Read the model definition and answer for the solid it produces. Units are mm, in the model's axes. Face numbers are marked on the shaded views. A direction names the side the tool comes from. Round coordinates to 2 decimals unless told otherwise and drop trailing zeros. Order: outer loops, then holes, each group sorted by start corner. A loop starts at its lowest first (then second) coordinate and runs counter-clockwise, first axis right, second up. Notation, with made-up numbers: (67.5, 10) -> (119.5, 10) arc R6 cw to (119.5, 14) -> close; hole circle Ø1 at (88, 74). An arc over 180 degrees is marked (long way). Answer as a JSON object with one key per item and string values. Group by question number.
Item 1: Consider probe 1 along X at (y, z) = (2.5, 4); probe 2 along Z at (x, y) = (0.75, 1.95); probe 3 along Y at (x, z) = (3, 7.25). Determine where each line is inside the solid, lowest interval first. Write a range as from..to.
Item 2: Section B-B, the plane z = 7.5 is taken. Write down the section's boundary in (x, y), plus the area to 3 significant figures.
Item 3: For the marked faces 1, 2, 3 and 4, determine the directions among +Z, -Z, +X, -X, +Y, -Y from which every point of the face is accessible in a straight line to the end or side of a thin tool.
Item 4: Given P1, Ø0.5, axis at y = 5, z = 2, coming from the +X side; P2, Ø1.4, axis at y = 4, z = 6, coming from the -X side, each flat-ended and moving along its own axis, determine where each tip first touches the part or whether it passes through.
Item 5: Section A-A, the plane y = 4.2 is taken. Write down the section's boundary in (x, z).
Item 6: Section D-D, the plane x = -3.5 is taken. Write down the section's boundary in (y, z), plus the area to 3 significant figures.
Item 7: The mould has two halves that part along Z. Classify the marked faces 5, 6, 7 and 8: pulls with the +Z half, pulls with the -Z half, needs draft (parallel to the pull), parting line crosses it, or undercut.
Item 8: Section C-C, the plane y = 1.4 is taken. Write down the section's boundary in (x, z), plus the area to 3 significant figures.
from build123d import *

# Parameters (mm, degrees)
BOSS_EXTRUDE1_DEPTH = 8
SKETCH2_R           = 2
CUT_EXTRUDE1_DEPTH  = 8
CUT_EXTRUDE2_DEPTH  = 1.75


with BuildPart() as part:
    # Sketch1 → Boss-Extrude1 (new body)
    with BuildSketch(Plane.XY):
        Polygon((0, 5.25), (0, 0), (6.25, 0), (8, 1.75), (8, 3.5), (4.1, 3.5), (4.1, 5.25), align=None)
    extrude(amount=BOSS_EXTRUDE1_DEPTH)

    # Mirror1: part across plane


with BuildPart() as part_1:
    add(part.part)
    add(part.part.mirror(Plane(origin=(0, 0, 0), x_dir=(0, 0, 1), z_dir=(1, 0, 0))))

    # Sketch2 → Cut-Extrude1 (cut)
    with BuildSketch(Plane(origin=(0, 5.25, 0), x_dir=(1, 0, 0), z_dir=(0, 1, 0))):
        with Locations(Location((0, -4, 0), (0, 0, 270))):
            Circle(SKETCH2_R)
    extrude(amount=-CUT_EXTRUDE1_DEPTH, mode=Mode.SUBTRACT)

    # Sketch3 → Cut-Extrude2 (cut)
    with BuildSketch(Plane(origin=(0, 5.25, 0), x_dir=(1, 0, 0), z_dir=(0, 1, 0))):
        with BuildLine():
            ThreePointArc((4.1, -4), (2.864000698, -6.834350716), (0, -8))
            Line((0, -8), (4.1, -8))
            Line((4.1, -8), (4.1, -4))
        make_face()
        with BuildLine():
            Line((-4.1, 0), (-4.1, -4.1))
            ThreePointArc((-4.1, -4.1), (-2.899137803, -1.200862197), (0, 0))
            Line((0, 0), (-4.1, 0))
        make_face()
    extrude(amount=-CUT_EXTRUDE2_DEPTH, mode=Mode.SUBTRACT)


solid = part_1.part
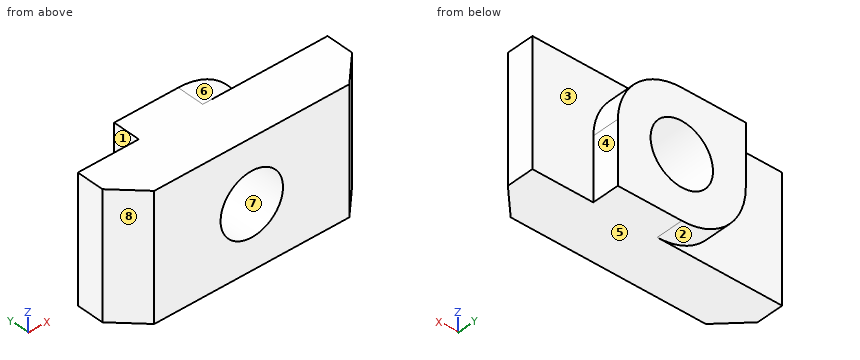
Values found:
{
 "1": {"probe 1": "-8..-2, 2..8", "probe 2": "0..2.15, 5.85..8", "probe 3": "0..3.5"},
 "2": {"outline": "(-8, 1.75) -> (-6.25, 0) -> (6.25, 0) -> (8, 1.75) -> (8, 3.5) -> (1.96, 3.5) -> (1.96, 5.25) -> (-4.1, 5.25) -> (-4.1, 3.5) -> (-8, 3.5) -> close", "area": "63.5 mm2"},
 "3": {"face 1": "+Z, -Z, -X, +Y", "face 2": "-Z, -X, +Y", "face 3": "+Z, +X, +Y", "face 4": "+Z, -Z, +X, +Y"},
 "4": {"P1": "x = 4.1", "P2": "x = -8"},
 "5": {"outline": "(-4.1, 4.1) arc R4.1 ccw to (0, 0) -> (4.1, 0) -> (4.1, 4) arc R4.1 ccw to (0, 8) -> (-4.1, 8) -> close; hole circle Ø4 at (0, 4)"},
 "6": {"outline": "(0, 0) -> (3.5, 0) -> (3.5, 1.96) -> (5.25, 1.96) -> (5.25, 8) -> (0, 8) -> close", "area": "38.6 mm2"},
 "7": {"face 5": "pulls with the -Z half", "face 6": "pulls with the +Z half", "face 7": "undercut", "face 8": "needs draft"},
 "8": {"outline": "(-7.65, 0) -> (7.65, 0) -> (7.65, 8) -> (-7.65, 8) -> close; hole circle Ø4 at (0, 4)", "area": "110 mm2"}
}
